Part model, mm, in its own coordinate system. Coordinates: 2 decimals unless noted, no trailing zeros. Order: outer loops, then holes, each group sorted by start corner. A loop starts at its lowest first (then second) coordinate and runs counter-clockwise, first axis right, second up.
Autodesk Inventor part; units mm, degrees
ref_plane "YZ Plane" through (0, 0, 0) normal (1, 0, 0) x (0, 1, 0)
ref_plane "XZ Plane" through (0, 0, 0) normal (0, 1, 0) x (-1, 0, 0)
ref_plane "XY Plane" through (0, 0, 0) normal (0, 0, 1) x (1, 0, 0)
sketch "Sketch1" plane through (0, 0, 0) normal (0, 1, 0) x (-1, 0, 0)
  line L0 (0, 0) -> (-362.1532, 0)
  line L1 (0, 0) -> (-362.1532, 0) construction
  line L2 (0, 0) -> (-362.1532, 0) construction
  line L3 (0, 25.4) -> (-362.1532, 25.4)
  line L4 (-362.1532, -25.4) -> (0, -25.4)
  arc A0 (0, -25.4) -> (0, 25.4) centre (0, 0) ccw
  arc A1 (-362.1532, 25.4) -> (-362.1532, -25.4) centre (-362.1532, 0) ccw
  circle A2 centre (0, 0) radius 14.2875
  circle A3 centre (-362.1532, 0) radius 14.2875
  circle A4 centre (-311.3532, 0) radius 3.175
  circle A5 centre (-298.6532, 0) radius 3.175
  circle A6 centre (-285.9532, 0) radius 3.175
  circle A7 centre (-273.2532, 0) radius 3.175
  circle A8 centre (-260.5532, 0) radius 3.175
  point P0 (-181.0766, 0)
  point P1 (-181.0766, 0)
  dimension "d0" = 362.1532
  dimension "d8" = 50.8
  dimension "d9" = 28.575
  dimension "d10" = 28.575
  dimension "d11" = 6.35
  dimension "d12" = 50.8
  dimension "d13" = 6.35
  dimension "d14" = 6.35
  dimension "d15" = 6.35
  dimension "d16" = 6.35
  dimension "d17" = 12.7
  dimension "d18" = 12.7
  dimension "d19" = 12.7
  dimension "d20" = 12.7
extrude "Extrusion1" add sketch "Sketch1" along normal blind 6.35
properties part number "4-bar intake (14.258) bar"
Q1. Mould opens along X. For faces 1 (the face through (-25.394, 3.131, 0.559)), 2 (the face through (184, 6.35, 0)), 3 (the face through (14.274, 3.131, -0.628)) say: pulls with the +X half, pulls with the -X half, needs draft (parallel to the pull), parting line crosses it, or undercut.
Results list:
face 1: pulls with the -X half
face 2: needs draft
face 3: undercut
Q2. Cut at B-B on z = 7. Write the cut outline in (x, y).
Results list:
outline: (-24.42, 0) - (-12.46, 0) - (-12.46, 6.35) - (-24.42, 6.35) - close; (12.46, 0) - (349.7, 0) - (349.7, 6.35) - (12.46, 6.35) - close; (374.61, 0) - (386.57, 0) - (386.57, 6.35) - (374.61, 6.35) - close
Q3. Cut at A-A on y = 4.25. Count the separate pieces of the cut face and the enclosed holes in it, and give its area (3 significant figures).
Results list:
separate pieces: 1
enclosed holes: 7
area: 19,000 mm2
Q4. Cut at C-C on z = -18.5. Write the cut outline in (x, y).
Results list:
outline: (-17.4, 0) - (379.56, 0) - (379.56, 6.35) - (-17.4, 6.35) - close
Q5. Pin check, flat tips, straight feed: pin 1 Ø3 at (y, z) = (1, 9) entering from -X; pin 2 Ø3 at (y, z) = (3, 2) entering from -X. Stop position of each tip, or through.
Results list:
pin 1: stops at x = -24.27
pin 2: stops at x = -25.4
Q6. Wall check: line 1 along X through (y, z) = (4.75, -7); line 2 along X through (y, z) = (4.75, -13); line 3 along Z through (x, y) = (0, 2.5). Give the ranges that are in metal, low to high.
Results list:
line 1: x = -24.42 to -12.46, 12.46 to 349.7, 374.61 to 386.57
line 2: x = -21.82 to -5.93, 5.93 to 356.23, 368.08 to 383.97
line 3: z = -25.4 to -14.29, 14.29 to 25.4
